from build123d import *

# Parameters (mm, degrees)
CYLINDER_R     = 1.75
CYLINDER_DEPTH = 5
EXTRUDE_DEPTH  = 28


with BuildPart() as cylindre:
    # Cylinder → Cylinder (new body)
    with BuildSketch(Plane(origin=(0, 3, 14), x_dir=(0, 0, -1), z_dir=(1, 0, 0))):
        Circle(CYLINDER_R)
    extrude(amount=CYLINDER_DEPTH)


with BuildPart() as cut:
    # Sketch → Extrude (new body)
    with BuildSketch(Plane.XY):
        Polygon((0, 0), (0, 5), (3, 8), (5, 8), (5, 0), align=None)
    extrude(amount=EXTRUDE_DEPTH)

    # Cut: cut Cylindre
    add(cylindre.part, mode=Mode.SUBTRACT)


solid = cut.part
Geometry check sheet. Reference: the model listing, model coordinates, mm. Round coordinates to 2 decimals unless told otherwise and drop trailing zeros. Loops run counter-clockwise (first coordinate to the right, second up) from the corner with the lowest first, then second, coordinate; pieces in that order, holes last.
Item 1: Thickness scan on line 1 (Y direction, x = 3.25, z = 14); line 2 (X direction, y = 6.25, z = 26.5); line 3 (Y direction, x = 2.25, z = 14). Record the ranges inside material, lowest first.
Item 2: Mould release check, pull along Y, two halves, no side actions. Record for faces 1 (the cylindrical face through (2.46, 1.45, 13.19)), 2 (the flat face through (1, 6, 14)), 3 (the flat face through (5, 5, 14)), 4 (the flat face through (3, 0, 14)): pulls with the +Y half, pulls with the -Y half, needs draft (parallel to the pull), parting line crosses it, or undercut.
Item 3: Cross-section at C-C on x = 1.2. Record the boundary of the cut face in (y, z).
Item 4: Cross-section at B-B on y = 3. Record the boundary of the cut face in (x, z).
Item 5: Cross-section at D-D on z = 19.25. Record the boundary of the cut face in (x, y), then the cut area to 3 significant figures.
Item 6: Cross-section at A-A on z = 14. Record the boundary of the cut face in (x, y), then the cut area to 3 significant figures.
Answer sheet:
1. line 1: y = 0 to 1.25, 4.75 to 8
1. line 2: x = 1.25 to 5
1. line 3: y = 0 to 1.25, 4.75 to 7.25
2. face 1: undercut
2. face 2: pulls with the +Y half
2. face 3: needs draft
2. face 4: pulls with the -Y half
3. outline: (0, 0) - (6.2, 0) - (6.2, 28) - (0, 28) - close; hole circle Ø3.5 at (3, 14)
4. outline: (0, 0) - (5, 0) - (5, 12.25) - (0, 12.25) - close; (0, 15.75) - (5, 15.75) - (5, 28) - (0, 28) - close
5. outline: (0, 0) - (5, 0) - (5, 8) - (3, 8) - (0, 5) - close
5. area: 35.5 mm2
6. outline: (0, 0) - (5, 0) - (5, 1.25) - (0, 1.25) - close; (0, 4.75) - (5, 4.75) - (5, 8) - (3, 8) - (0, 5) - close
6. area: 18.0 mm2
